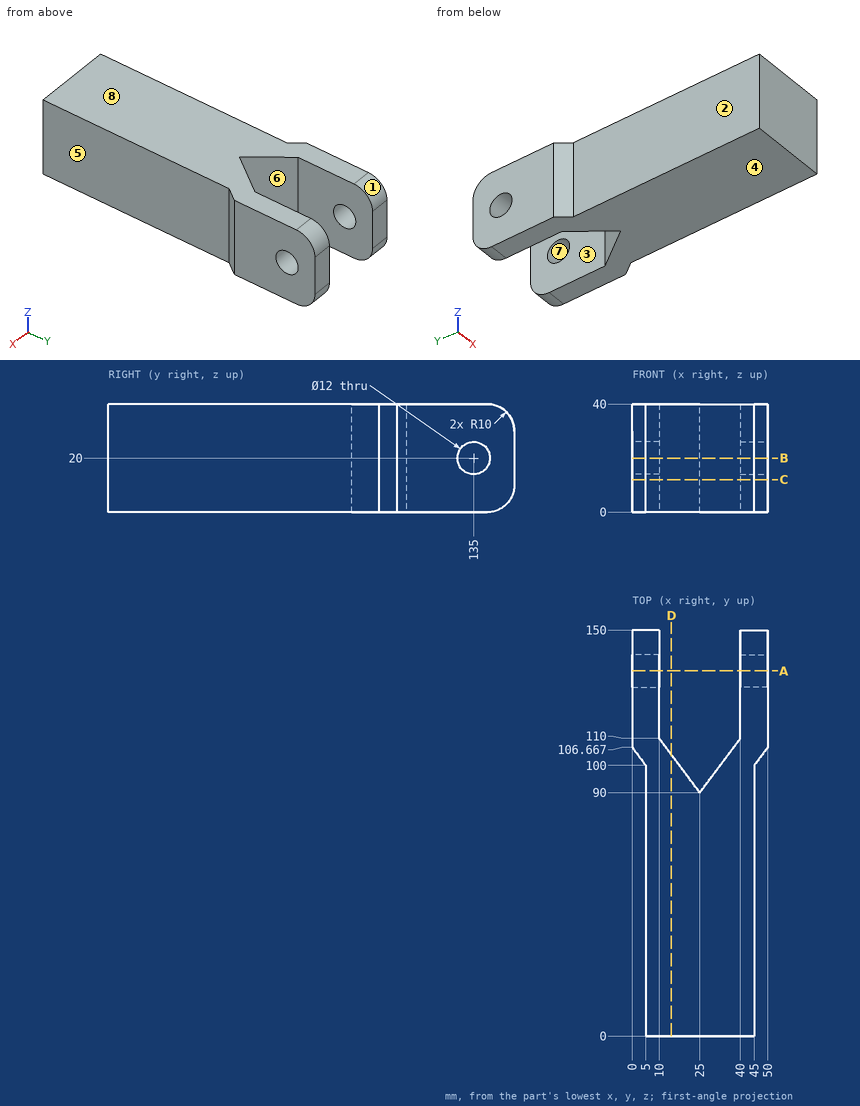
Source: three-view drawing plus pictorial views. Frame: mm from the lowest corner of the part. A direction names the side the tool comes from. Coordinates: 2 decimals unless noted, no trailing zeros. Order: outer loops, then holes, each group sorted by start corner. A loop starts at its lowest first (then second) coordinate and runs counter-clockwise, first axis right, second up.
1) Section B-B (z = 20). Return loops of the section in (x, y).
Result sheet:
outline: (0, 106.67) - (5, 100) - (5, 0) - (45, 0) - (45, 100) - (50, 106.67) - (50, 129) - (40, 129) - (40, 110) - (25, 90) - (10, 110) - (10, 129) - (0, 129) - close; (0, 141) - (10, 141) - (10, 150) - (0, 150) - close; (40, 141) - (50, 141) - (50, 150) - (40, 150) - close
2) First-contact query: P1, Ø1.5, axis at x = 17.5, z = 29, coming from the -Y side; P2, Ø10, axis at y = 84, z = 30, coming from the -X side; P3, Ø3, axis at y = 18.5, z = 31.5, coming from the +X side; P4, Ø6, axis at x = 36.5, z = 32.5, coming from the +Y side (1 decimal). Flat tips, straight axial feed; report the tip coordinate or a pass-through.
Result sheet:
P1: stops at y = 0
P2: stops at x = 5
P3: stops at x = 45
P4: stops at y = 109.3
3) Draft query along Y for the marked faces 6, 7 and 8. Return one class per face: released by +Y, released by -Y, zero draft, split by the parting line, or undercut.
Result sheet:
face 6: released by +Y
face 7: undercut
face 8: zero draft
4) Set-up query: the marked faces 1, 2, 3, 4 and 5. Return all of +Z, -Z, +X, -X, +Y, -Y with unobstructed straight access to the full face (end or side cutting, diameter ignored); none if empty.
Result sheet:
face 1: +Z, +X, -X, +Y
face 2: +Z, -Z, -X, -Y
face 3: +Z, -Z, +Y
face 4: -Z, +X, -X, +Y, -Y
face 5: +Z, -Z, +X, -Y
5) Section A-A (y = 135). Return loops of the section in (x, z), then the cut area to 3 significant figures.
Result sheet:
outline: (0, 0) - (10, 0) - (10, 14) - (0, 14) - close; (0, 26) - (10, 26) - (10, 40) - (0, 40) - close; (40, 0) - (50, 0) - (50, 14) - (40, 14) - close; (40, 26) - (50, 26) - (50, 40) - (40, 40) - close
area: 560 mm2
6) Section D-D (x = 14.5). Return loops of the section in (y, z).
Result sheet:
outline: (0, 0) - (104, 0) - (104, 40) - (0, 40) - close
7) Section C-C (z = 12). Return loops of the section in (x, y).
Result sheet:
outline: (0, 106.67) - (5, 100) - (5, 0) - (45, 0) - (45, 100) - (50, 106.67) - (50, 150) - (40, 150) - (40, 110) - (25, 90) - (10, 110) - (10, 150) - (0, 150) - close
8) Ray query, probe 1 along Z at (x, y) = (43, 135); probe 2 along X at (y, z) = (144.5, 11); probe 3 along X at (y, z) = (63, 37.5). Return the intervals inside material, ascending.
Result sheet:
probe 1: z = 0 to 14, 26 to 40
probe 2: x = 0 to 10, 40 to 50
probe 3: x = 5 to 45
